Print and shaded views of the part. All mm, measured from the part's lowest x, y and z. Round coordinates to 2 decimals unless told otherwise and drop trailing zeros. Loops run counter-clockwise (first coordinate to the right, second up) from the corner with the lowest first, then second, coordinate; pieces in that order, holes last. Notation, with made-up numbers: (-26.75, 14.25) - (-7.75, 14.25) arc R37 cw to (-7.75, 53.25) - close; hole circle Ø2 at (-14.75, 69). An arc over 180 degrees is marked (long way). Use one line per item in the form item = value.
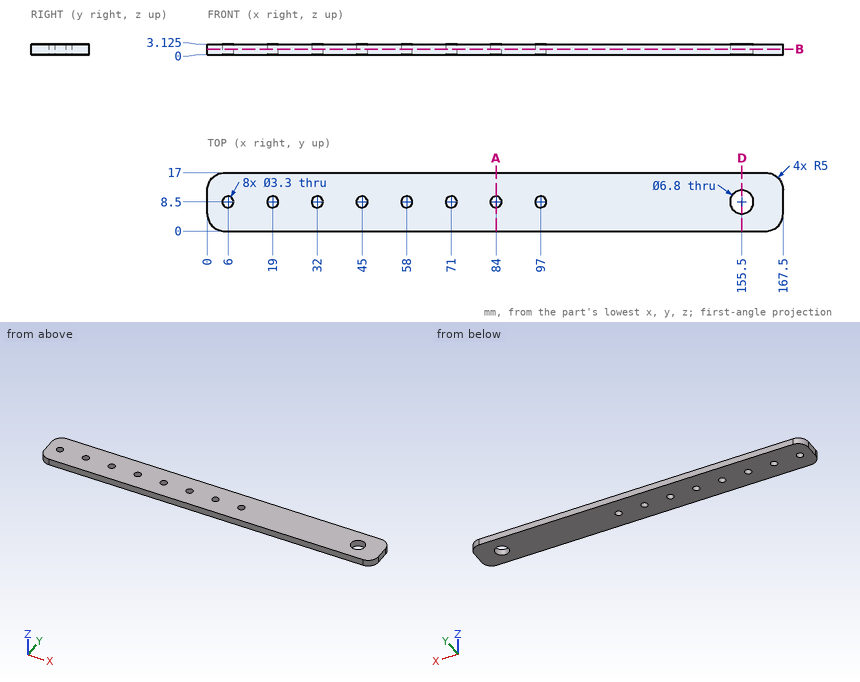
1) Slice it at D-D (x = 155.5). Write the cut outline in (y, z) (3 decimals).
Report:
outline = (0, 0) - (5.1, 0) - (5.1, 3.125) - (0, 3.125) - close; (11.9, 0) - (17, 0) - (17, 3.125) - (11.9, 3.125) - close
2) Slice it at A-A (x = 84). Write the cut outline in (y, z) (3 decimals).
Report:
outline = (0, 0) - (6.85, 0) - (6.85, 3.125) - (0, 3.125) - close; (10.15, 0) - (17, 0) - (17, 3.125) - (10.15, 3.125) - close
3) Slice it at B-B (z = 1.6). State how many separate pieces and enclosed holes the cut face has, plus the area to 3 significant figures.
Report:
separate_pieces = 1
enclosed_holes = 9
area = 2,720 mm^2
4) Flat gauge pins, fed straight in: pin 1 (1.5 mm diameter, centred on x = 114, z = 1.5, fed in from -Y); pin 2 (3 mm diameter, centred on x = 19, y = 8.5, fed in from +Z). Where does each tip first touch, or does it go through?
Report:
pin_1 = 0
pin_2 = through
5) Drill centre lines: probe 1 along Y at (x, z) = (58, 2); probe 2 along X at (y, z) = (4.75, 2.8); probe 3 along X at (y, z) = (11.5, 2.95). Where is each one in solid material? Low to high.
Report:
probe_1 = 0 to 6.85, 10.15 to 17
probe_2 = 0.01 to 167.49
probe_3 = 0 to 153.9, 157.1 to 167.5
